Autodesk Inventor part; units mm, degrees
ref_plane "YZ Plane" through (0, 0, 0) normal (1, 0, 0) x (0, 1, 0)
ref_plane "XZ Plane" through (0, 0, 0) normal (0, 1, 0) x (-1, 0, 0)
ref_plane "XY Plane" through (0, 0, 0) normal (0, 0, 1) x (1, 0, 0)
sketch "スケッチ3" plane through (0, 0, 0) normal (0, 0, 1) x (1, 0, 0)
  line L0 (60, -99.3436) -> (-60, -99.3436)
  line L1 (-60, -99.3436) -> (-60, 99.3436)
  line L2 (-60, 99.3436) -> (60, 99.3436)
  line L3 (60, 99.3436) -> (60, -99.3436)
  line L4 (60, -99.3436) -> (-60, 99.3436) construction
  line L5 (-60, -99.3436) -> (60, 99.3436) construction
  point P0 (0, 0)
  dimension "d25" = 120
extrude "押し出し1" add sketch "スケッチ3" against normal blind 3
sketch "スケッチ4" plane through (0, 0, 0) normal (0, 0, 1) x (1, 0, 0)
  line L0 (0, 45.0711) -> (68.3595, 45.0711)
  line L1 (68.3595, 45.0711) -> (-74.3824, 45.0711)
  line L2 (-74.3824, 45.0711) -> (108.1656, 45.0711)
  line L3 (108.1656, 45.0711) -> (108.1656, 129.4154)
  line L4 (108.1656, 129.4154) -> (-74.3824, 129.4154)
  line L5 (-74.3824, 129.4154) -> (-74.3824, 45.0711)
  point P0 (0, 0)
extrude "押し出し4" cut sketch "スケッチ4" against normal blind 10
sketch "スケッチ13" plane through (0, 0, 0) normal (0, 0, 1) x (1, 0, 0)
  circle A0 centre (0, 0) radius 7.5
  circle A1 centre (0, 0) radius 32.5
  circle A2 centre (31.7707, 6.8465) radius 25
  circle A3 centre (31.7707, 6.8465) radius 7.5
  circle A4 centre (31.7707, 6.8465) radius 32.5
  circle A5 centre (28.5436, -25.4929) radius 25
  circle A6 centre (28.5436, -25.4929) radius 20
  circle A7 centre (28.5436, -25.4929) radius 60
  circle A8 centre (0, -78.2685) radius 40
  circle A9 centre (0, -78.2685) radius 50
  circle A10 centre (31.7707, 6.8465) radius 5
  circle A11 centre (28.5436, -25.4929) radius 9.5
  circle A12 centre (0, -78.2685) radius 9.5
  dimension "d87" = 65
  dimension "d89" = 65
  dimension "d91" = 120
  dimension "d86" = 15
  dimension "d88" = 15
  dimension "d90" = 40
  dimension "d92" = 100
  dimension "d96" = 10
  dimension "d97" = 19
  dimension "d98" = 19
extrude "押し出し16" cut sketch "スケッチ13" against normal blind 10 contours A10 A1 | A1 A10 | A11 A1 A2 | A2 A1 A4 A11 | A4 A1 A11 | A2 A11 A4 A1 | A1 A11 A2 | A4 A11 A1 | A12 A7 | A7 A12
sketch "スケッチ14" plane through (0, 0, 0) normal (0, 0, 1) x (1, 0, 0)
  point P0 (0, 0)
sketch "スケッチ15" plane through (0, 0, 0) normal (0, 0, 1) x (1, 0, 0)
  line L0 (-60, -99.3436) -> (-60, 45.0711)
  line L1 (60, 45.0711) -> (60, -99.3436)
  line L2 (-60, 45.0711) -> (60, 45.0711)
  line L3 (60, 45.0711) -> (60, -92.9289)
  line L4 (60, -92.9289) -> (-60, -92.9289)
  line L5 (-60, -92.9289) -> (-60, 45.0711)
  point P0 (0, 0)
  dimension "d101" = 138
extrude "押し出し17" cut sketch "スケッチ15" against normal blind 10 keep common part
sketch "スケッチ16" plane through (-60, 45.0711, 0) normal (0, 1, 0) x (1, 0, 0)
  line L0 (-11.4218, 21.1899) -> (145.405, 21.1899)
  line L1 (145.405, 21.1899) -> (145.405, -40.3361)
  line L2 (145.405, -40.3361) -> (-11.4218, -40.3361)
  line L3 (-11.4218, -40.3361) -> (-11.4218, 21.1899)
  point P0 (60, 0)
extrude "押し出し18" cut sketch "スケッチ16" against normal blind 10
sketch "スケッチ17" plane through (0, 0, 0) normal (0, 0, 1) x (1, 0, 0)
  circle A0 centre (31.7707, 6.8465) radius 5
  circle A1 centre (31.7707, 6.8465) radius 25
  circle A2 centre (28.5436, -25.4929) radius 9.5
  circle A3 centre (28.5436, -25.4929) radius 25
  circle A4 centre (55, -13) radius 2
  circle A5 centre (-55, -13) radius 2
  circle A6 centre (0, 29) radius 2
  point P0 (0, 0)
  point P1 (0, 0)
  dimension "d106" = 50
  dimension "d107" = 50
  dimension "d108" = 4
  dimension "d109" = 4
  dimension "d110" = 4
extrude "押し出し19" cut sketch "スケッチ17" against normal blind 10 contours A4 | A5 | A6
properties part number "板2" material "アルミニウム 6061"
Verification items for the finished model (mm, model axes). Round coordinates to 2 decimals unless told otherwise and drop trailing zeros. Loops run counter-clockwise (first coordinate to the right, second up) from the corner with the lowest first, then second, coordinate; pieces in that order, holes last. Notation, with made-up numbers: (71.5, -26.75) -> (124.5, -26.75) arc R17 ccw to (124.5, -16.75) -> close; hole circle Ø5 at (43, -26.5). An arc over 180 degrees is marked (long way). Answer as a JSON object with one key per item and string values.
Q1. Scan lines: line 1 (Y direction, x = 0, z = -1.3); line 2 (Y direction, x = -55, z = -2); line 3 (X direction, y = -71, z = -0.35). Record each from-to range of solid material in increasing order. Write a range as from..to.
Data:
{"line 1": "y = -92.93..-87.77, -68.77..27, 31..35.07", "line 2": "y = -92.93..-15, -11..35.07", "line 3": "x = -60..-6.12, 6.12..60"}
Q2. Section check B-B (x = 0). Record the boundary of the cut face in (y, z), then the cut area to 3 significant figures.
Data:
{"outline": "(-92.93, -3) -> (-87.77, -3) -> (-87.77, 0) -> (-92.93, 0) -> close; (-68.77, -3) -> (27, -3) -> (27, 0) -> (-68.77, 0) -> close; (31, -3) -> (35.07, -3) -> (35.07, 0) -> (31, 0) -> close", "area": "315 mm2"}
Q3. Section check A-A (y = -13). Record the boundary of the cut face in (x, z), then the cut area to 3 significant figures.
Data:
{"outline": "(-60, -3) -> (-57, -3) -> (-57, 0) -> (-60, 0) -> close; (-53, -3) -> (53, -3) -> (53, 0) -> (-53, 0) -> close; (57, -3) -> (60, -3) -> (60, 0) -> (57, 0) -> close", "area": "336 mm2"}
Q4. Draft check along Y on faces 1 (the flat face through (1, -92.929, -1)), 2 (the flat face through (60, -28, -1)), 3 (the cylindrical face through (5.11, -70.26, -1.48)). Enter one of: pulls with the +Y half, pulls with the -Y half, needs draft (parallel to the pull), parting line crosses it, or undercut.
Data:
{"face 1": "pulls with the -Y half", "face 2": "needs draft", "face 3": "undercut"}
Q5. Section check D-D (x = -55). Record the boundary of the cut face in (y, z), then the cut area to 3 significant figures.
Data:
{"outline": "(-92.93, -3) -> (-15, -3) -> (-15, 0) -> (-92.93, 0) -> close; (-11, -3) -> (35.07, -3) -> (35.07, 0) -> (-11, 0) -> close", "area": "372 mm2"}
Q6. Section check C-C (y = 29). Record the boundary of the cut face in (x, z).
Data:
{"outline": "(-60, -3) -> (-2, -3) -> (-2, 0) -> (-60, 0) -> close; (2, -3) -> (60, -3) -> (60, 0) -> (2, 0) -> close"}
